from build123d import *

# Parameters (mm, degrees)
SKETCH022_R  = 3.571875
PAD022_DEPTH = 55
SKETCH021_R  = 3.571875
PAD021_DEPTH = 55
SKETCH020_R  = 3.571875
PAD020_DEPTH = 30
PAD002_DEPTH = 12.7


with BuildPart() as body022:
    # Sketch022 → Pad022 (new body)
    with BuildSketch(Plane.XY):
        Circle(SKETCH022_R)
    extrude(amount=PAD022_DEPTH)


with BuildPart() as body022_1:
    # Body022 placement: moved
    add(body022.part.moved(Location((150, -6.35, 115))))


with BuildPart() as body021:
    # Sketch021 → Pad021 (new body)
    with BuildSketch(Plane.XY):
        Circle(SKETCH021_R)
    extrude(amount=PAD021_DEPTH)


with BuildPart() as body021_1:
    # Body021 placement: moved
    add(body021.part.moved(Location((100, -6.35, 115))))


with BuildPart() as body020:
    # Sketch020 → Pad020 (new body)
    with BuildSketch(Plane.XZ):
        Circle(SKETCH020_R)
    extrude(amount=PAD020_DEPTH)


with BuildPart() as body020_1:
    # Body020 placement: moved
    add(body020.part.moved(Location((25, 2, 149.369))))


with BuildPart() as braceupper:
    # Sketch002 → Pad002 (new body)
    with BuildSketch(Plane.XZ):
        with BuildLine():
            Line((-20, 110), (-20, 155))
            Line((-20, 155), (50, 155))
            Line((50, 155), (50, 110))
            Line((50, 110), (28.325, 110))
            ThreePointArc((28.325, 110), (15, 123.324967), (1.675, 110))
            Line((-20, 110), (1.675, 110))
        make_face()
    extrude(amount=PAD002_DEPTH)


with BuildPart() as braceupper_1:
    # Body002 placement: moved
    add(braceupper.part.moved(Location((10, 0, 10))))

    # Cut013: cut Body020
    add(body020_1.part, mode=Mode.SUBTRACT)


with BuildPart() as braceupper_2:
    # Cut013 placement: moved
    add(braceupper_1.part.moved(Location((100, 0, 0))))

    # Cut014: cut Body021
    add(body021_1.part, mode=Mode.SUBTRACT)

    # Cut015: cut Body022
    add(body022_1.part, mode=Mode.SUBTRACT)


with BuildPart() as braceupper_3:
    # Cut015 placement: moved
    add(braceupper_2.part.moved(Location((-100, 0, 0))))


solid = braceupper_3.part
Source: CAD feature listing. Evaluate the final solid. Frame: model axes, mm. Give positions to 0.01 mm unless a question says otherwise; leave off trailing zeros. Loops run counter-clockwise (first coordinate to the right, second up) from the corner with the lowest first, then second, coordinate; pieces in that order, holes last. Notation, with made-up numbers: (35, 10) -> (48, 10) arc R5 ccw to (48, 15) -> close; hole circle Ø4 at (1, 69.25). An arc over 180 degrees is marked (long way). Use a Markdown table: item, result. Add a question column.
1) Pull-direction query (Y, two-part tool) for faces 1 (the face through (46.43, -6.19, 142.18)), 2 (the face through (25, 0, 143)), 3 (the face through (60, -6, 143)); classes: +Y half, -Y half, draft (parallel to the pull), parting line (faces both ways), or undercut.
2) Section query B-B, the plane x = 0. Return the cut outline in (y, z).
3) Section query D-D, the plane z = 140. Return the cut outline in (x, y).
4) First-contact query: pin 1 (6.5 mm diameter, centred on x = 25, z = 149.369, fed in from -Y); pin 2 (1.5 mm diameter, centred on x = 26.5, y = -6.5, fed in from -Z). Flat tips, straight axial feed; report the tip coordinate or a pass-through.
5) Section query A-A, the plane y = -6.35. Return the cut outline in (x, z) (3 decimals), then the cut area to 3 significant figures.
6) Section query C-C, the plane z = 124. Return the cut outline in (x, y), then the cut area to 3 significant figures.
7) Line query: line 1 along X through (y, z) = (-6.35, 138); line 2 along Z through (x, y) = (25, -4.5); line 3 along X through (y, z) = (-7, 126). Output: solid intervals per line, ascending. Write a range as [from, to].
Numbers:
| question | item | result |
|---|---|---|
| 1 | face 1 | undercut |
| 1 | face 2 | +Y half |
| 1 | face 3 | draft |
| 2 | outline | (-12.7, 120) -> (-9.92, 120) -> (-9.92, 165) -> (-12.7, 165) -> close; (-2.78, 120) -> (0, 120) -> (0, 165) -> (-2.78, 165) -> close |
| 3 | outline | (-10, -12.7) -> (60, -12.7) -> (60, 0) -> (-10, 0) -> close; hole circle Ø7.14 at (0, -6.35); hole circle Ø7.14 at (50, -6.35) |
| 4 | pin 1 | passes through |
| 4 | pin 2 | stops at z = 133.13 |
| 5 | outline | (-10, 120) -> (-3.572, 120) -> (-3.572, 165) -> (-10, 165) -> close; (3.572, 120) -> (11.675, 120) arc R13.325 cw to (38.325, 120) -> (46.428, 120) -> (46.428, 165) -> (3.572, 165) -> close; (53.572, 120) -> (60, 120) -> (60, 165) -> (53.572, 165) -> close; hole circle Ø7.144 at (25, 149.369) |
| 5 | area | 2,190 mm2 |
| 6 | outline | (-10, -12.7) -> (12.29, -12.7) -> (12.29, 0) -> (-10, 0) -> close; (37.71, -12.7) -> (60, -12.7) -> (60, 0) -> (37.71, 0) -> close; hole circle Ø7.14 at (0, -6.35); hole circle Ø7.14 at (50, -6.35) |
| 6 | area | 486 mm2 |
| 7 | line 1 | x = [-10, -3.57], [3.57, 46.43], [53.57, 60] |
| 7 | line 2 | z = [133.32, 145.8], [152.94, 165] |
| 7 | line 3 | x = [-10, -3.51], [3.51, 13.1], [36.9, 46.49], [53.51, 60] |
